from build123d import *

# Parameters (mm, degrees)
F0_W     = 250
F0_H     = 40
F1_DEPTH = 150
F2_T     = -2.5


# Not quite as in the source:
# - the program builds the solid bodies; features that only make, move or delete a surface that nothing else refers to are left out


with BuildPart() as f1:
    # F0 (on Front) → F1 (new body)
    with BuildSketch(Plane.XZ):
        with Locations((-125, 20)):
            Rectangle(F0_W, F0_H)
    extrude(amount=-F1_DEPTH)

    # F2
    f2_openings = [f1.faces().sort_by_distance(p)[0] for p in [
        (-125, 75, 0),
    ]]
    offset(amount=F2_T, openings=f2_openings)


solid = f1.part
Model file for the job. Use its own axes, mm. A direction names the side the tool comes from. Give positions to 0.01 mm unless a question says otherwise; leave off trailing zeros. Loops run counter-clockwise (first coordinate to the right, second up) from the corner with the lowest first, then second, coordinate; pieces in that order, holes last.
1) Saw through at A-A (z = 11.5). Write the cut outline in (x, y).
2) Saw through at C-C (y = 102.5). Write the cut outline in (x, z), plus the area to 4 significant figures.
3) Pull direction Y, two halves, no side cores. Call faces 3 (the flat face through (0, 74, 20)), 4 (the flat face through (-127, 74, 37.5)), 5 (the flat face through (-247.5, 74, 18)), 6 (the flat face through (-127, 150, 20)): +Y half, -Y half, draft (parallel to the pull), parting line (faces both ways), or undercut.
4) Wall check: line 1 (Y direction, x = -58.5, z = 31); line 2 (X direction, y = 91, z = 32.5); line 3 (Z direction, x = -186.5, y = 49). Give the ranges that are in metal, low to high.
5) Tool access for faces 1 (the flat face through (-127, 2.5, 19)), 2 (the flat face through (-126, 2, 0)): list every direction of +Z, -Z, +X, -X, +Y, -Y with a clear straight run to the whole face (end or side of a thin tool).
6) Saw through at B-B (x = -127). Write the cut outline in (y, z).
7) Flat gauge pins, fed straight in: pin 1 Ø1 at (y, z) = (73.5, 17.5) entering from +X; pin 2 Ø8 at (x, y) = (-104.5, 26.5) entering from -Z. Where does each tip first touch, or does it go through?
Answer block:
1. outline: (-250, 0) - (0, 0) - (0, 150) - (-250, 150) - close; hole (-247.5, 2.5) - (-2.5, 2.5) - (-2.5, 147.5) - (-247.5, 147.5) - close
2. outline: (-250, 0) - (-247.5, 0) - (-247.5, 37.5) - (-2.5, 37.5) - (-2.5, 0) - (0, 0) - (0, 40) - (-250, 40) - close
2. area: 812.5 mm2
3. face 3: draft
3. face 4: undercut
3. face 5: undercut
3. face 6: +Y half
4. line 1: y = 0 to 2.5, 147.5 to 150
4. line 2: x = -250 to -247.5, -2.5 to 0
4. line 3: z = 37.5 to 40
5. face 1: -Z
5. face 2: -Z, +X, -X, +Y, -Y
6. outline: (0, 0) - (2.5, 0) - (2.5, 37.5) - (147.5, 37.5) - (147.5, 0) - (150, 0) - (150, 40) - (0, 40) - close
7. pin 1: stops at x = 0
7. pin 2: stops at z = 37.5
